Here's how the part is built. I have some questions about the finished solid (model axes, mm). Face numbers are marked on the shaded views. A direction names the side the tool comes from. Coordinates: 2 decimals unless noted, no trailing zeros. Loops run counter-clockwise (first coordinate to the right, second up) from the corner with the lowest first, then second, coordinate; pieces in that order, holes last.
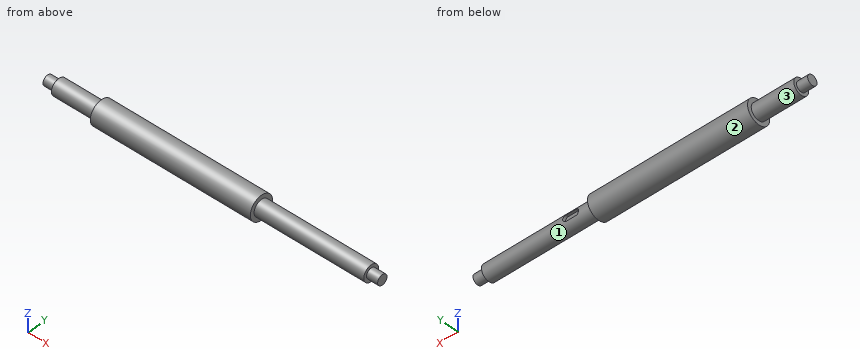
```python
from build123d import *

# Parameters (mm, degrees)
SKETCH1_R           = 9.525
BOSS_EXTRUDE1_DEPTH = 266.7
SKETCH4_R           = 9.525
SKETCH4_R_2         = 6.35
CUT_EXTRUDE3_DEPTH  = 42.799
SKETCH5_R           = 6.35
SKETCH5_R_2         = 4
CUT_EXTRUDE4_DEPTH  = 8.89
CUT_EXTRUDE5_START  = -96.3295
SKETCH6_R           = 9.525
SKETCH6_R_2         = 6.35
CUT_EXTRUDE5_DEPTH  = 96.3295
CUT_EXTRUDE6_DEPTH  = 2.3876


with BuildPart() as part:
    # Sketch1 → Boss-Extrude1 (new body)
    with BuildSketch(Plane(origin=(0, 0, 0), x_dir=(0, 0, -1), z_dir=(1, 0, 0))):
        Circle(SKETCH1_R)
    extrude(amount=BOSS_EXTRUDE1_DEPTH)

    # Sketch4 → Cut-Extrude3 (cut)
    with BuildSketch(Plane.ZY):
        Circle(SKETCH4_R)
        Circle(SKETCH4_R_2, mode=Mode.SUBTRACT)
    extrude(amount=-CUT_EXTRUDE3_DEPTH, mode=Mode.SUBTRACT)

    # Sketch5 → Cut-Extrude4 (cut)
    with BuildSketch(Plane.ZY):
        Circle(SKETCH5_R)
        Circle(SKETCH5_R_2, mode=Mode.SUBTRACT)
    cut_extrude4 = extrude(amount=-CUT_EXTRUDE4_DEPTH, mode=Mode.SUBTRACT)

    # Sketch6 → Cut-Extrude5 (cut)
    with BuildSketch(Plane(origin=(266.7, 0, 0), x_dir=(0, 0, -1), z_dir=(1, 0, 0)).offset(CUT_EXTRUDE5_START)):
        with Locations(Location((0, 0, 0), (0, 0, 180))):
            Circle(SKETCH6_R)
        with Locations(Location((0, 0, 0), (0, 0, 180))):
            Circle(SKETCH6_R_2, mode=Mode.SUBTRACT)
    extrude(amount=CUT_EXTRUDE5_DEPTH, mode=Mode.SUBTRACT)

    # Mirror1: Cut-Extrude4 across plane
    add(cut_extrude4.mirror(Plane.ZY.offset(-133.35)), mode=Mode.SUBTRACT)

    # Sketch7 → Cut-Extrude6 (cut)
    with BuildSketch(Plane(origin=(0, 6.35, 0), x_dir=(1, 0, 0), z_dir=(0, 1, 0))):
        with BuildLine():
            Line((182.7911, 2.38125), (190.7286, 2.38125))
            ThreePointArc((190.7286, 2.38125), (193.10985, 0), (190.7286, -2.38125))
            Line((190.7286, -2.38125), (182.7911, -2.38125))
            ThreePointArc((182.7911, -2.38125), (180.40985, 0), (182.7911, 2.38125))
        make_face()
    extrude(amount=-CUT_EXTRUDE6_DEPTH, mode=Mode.SUBTRACT)


solid = part.part
```
1. For pin 1 (6 mm diameter, centred on y = -6.5, z = 7, fed in from -X); pin 2 (5 mm diameter, centred on x = 27.5, y = 4, fed in from -Z); pin 3 (1 mm diameter, centred on x = 115.5, z = -5.5, fed in from +Y), each with a flat end and sliding along its axis, tell me the tip position at first contact or that it passes through.
2. I need wall thicknesses on line 1 along Z through (x, y) = (173, 0.5); line 2 along X through (y, z) = (-4.5, 7.25); line 3 along Z through (x, y) = (12, 3.5). Which ranges of each line are inside material? Lowest first, please.
3. I want a section at C-C (x = 141.5). Please give me the cut outline in (y, z) (3 decimals), then the cut area to 3 significant figures.
4. On a 3-axis mill with a long thin cutter (end or side, diameter ignored), from which of +Z, -Z, +X, -X, +Y, -Y can I reach the whole of each face in a straight line? I mean the marked faces 1, 2 and 3. Say none if no direction works.
Response values:
1. pin 1: stops at x = 42.8
1. pin 2: stops at z = -6.17
1. pin 3: stops at y = 8.11
2. line 1: z = -6.33 to 6.33
2. line 2: x = 42.8 to 170.37
2. line 3: z = -5.3 to 5.3
3. outline: circle Ø19.05 at (0, 0)
3. area: 285 mm2
4. face 1: +X
4. face 2: +X, -X
4. face 3: -X
